The model under review builds one solid part; all positions refer to its coordinate system, in mm. A direction names the side the tool comes from. Coordinates: 2 decimals unless noted, no trailing zeros. Loops run counter-clockwise (first coordinate to the right, second up) from the corner with the lowest first, then second, coordinate; pieces in that order, holes last. Notation, with made-up numbers: (55, -37.75) - (95, -37.75) arc R20 cw to (95, -30.75) - close; hole circle Ø4 at (69, -3.5). An arc over 180 degrees is marked (long way). Use a Markdown table: item, result. Add a question column.
1) Clearance check with flat-ended pins moving along their axes: pin 1 (1.5 mm diameter, centred on x = -10, y = 22, fed in from +Z); pin 2 (2 mm diameter, centred on y = 10, z = 2, fed in from -X); pin 3 (3 mm diameter, centred on x = -2, z = 0.5, fed in from -Y). State where each tip first meets the part, or that it passes through.
2) The part is to be moulded in two halves that separate along X. For faces 4 (the cylindrical face through (-3, 0, 4)), 5 (the cylindrical face through (1.27, -0.97, 0.99)), 6 (the flat face through (2, 16, 4)), 7 (the cylindrical face through (-12, 24, 1)), say which applies: pulls with the +X half, pulls with the -X half, needs draft (parallel to the pull), parting line crosses it, or undercut.
3) Add section A-A, the plane y = 21. Give the boundary of the cut face in (x, z), and give its area (3 significant figures).
4) Add section B-B, the plane x = 0. Give the boundary of the cut face in (y, z), and give its area (3 significant figures).
5) Add section C-C, the plane z = 1.6. Give the boundary of the cut face in (x, y).
6) Add section D-D, the plane y = 0. Give the boundary of the cut face in (x, z), and give its area (3 significant figures).
7) To check wall thickness, follow L1, parallel to Z at x = -4, y = 14.5; L2, parallel to Y at x = -4, z = 2.55; L3, parallel to Y at x = -4.25, z = 0.9. State the ranges of each line that lie inside material, in increasing order. Write a range as [from, to].
8) For faces 1 (the flat face through (-1.3, -1.3, 2)), 2 (the cylindrical face through (6.89, 22.01, 1.48)), 3 (the flat face through (-2, 16, 4)), list the 3-axis set-ups (+Z, -Z, +X, -X, +Y, -Y) from which the entire face can be reached by the end or side of a thin tool; tool diameter is ignored.
```python
from build123d import *
from build123d.topology import SkipClean

# Parameters (mm, degrees)
SZKIC1_R                    = 2.75
SZKIC1_R_2                  = 1.5
DODANIE_WYCI_GNI_CIE1_DEPTH = 3
SZKIC2_R                    = 6.131623165
SZKIC2_R_2                  = 2.75
DODANIE_WYCI_GNI_CIE2_DEPTH = 3
SZKIC3_R                    = 3
SZKIC3_R_2                  = 1.6
DODANIE_WYCI_GNI_CIE3_DEPTH = 2
SZKIC4_W                    = 4
SZKIC4_H                    = 20.653159846
DODANIE_WYCI_GNI_CIE4_DEPTH = 2
SZKIC6_R                    = 3
WYTNIJ_WYCI_GNI_CIE1_DEPTH  = 4


with BuildPart() as part:
    # Szkic1 → Dodanie-wyciągnięcie1 (new body)
    with BuildSketch(Plane.XY):
        with BuildLine():
            Line((-8, 26), (8, 26))
            ThreePointArc((8, 26), (12.044264582, 23.940055101), (12.756144284, 19.457569598))
            Line((12.756144284, 19.457569598), (5.832576894, -1.891520397))
            ThreePointArc((5.832576894, -1.891520397), (0, -6.131623165), (-5.832576894, -1.891520397))
            Line((-5.832576894, -1.891520397), (-12.756144284, 19.457569598))
            ThreePointArc((-12.756144284, 19.457569598), (-12.044264582, 23.940055101), (-8, 26))
        make_face()
        Circle(SZKIC1_R, mode=Mode.SUBTRACT)
        with Locations((8, 21)):
            Circle(SZKIC1_R_2, mode=Mode.SUBTRACT)
        with Locations((-8, 21)):
            Circle(SZKIC1_R_2, mode=Mode.SUBTRACT)
    extrude(amount=DODANIE_WYCI_GNI_CIE1_DEPTH)

    # Szkic2 → Dodanie-wyciągnięcie2 (add)
    with BuildSketch(Plane.XY.offset(3)):
        with Locations(Location((0, 0, 0), (0, 0, 197.968018337))):
            Circle(SZKIC2_R)
        Circle(SZKIC2_R_2, mode=Mode.SUBTRACT)
    extrude(amount=DODANIE_WYCI_GNI_CIE2_DEPTH)

    # Szkic3 → Dodanie-wyciągnięcie3 (add)
    with BuildSketch(Plane(origin=(0, 0, 0), x_dir=(-1, 0, 0), z_dir=(0, 0, -1))):
        Circle(SZKIC3_R)
        Circle(SZKIC3_R_2, mode=Mode.SUBTRACT)
    extrude(amount=-DODANIE_WYCI_GNI_CIE3_DEPTH)

    # Szkic4 → Dodanie-wyciągnięcie4 (add)
    with BuildSketch(Plane.XY.offset(3)):
        with Locations((0, 15.673420077)):
            Rectangle(SZKIC4_W, SZKIC4_H)
    extrude(amount=DODANIE_WYCI_GNI_CIE4_DEPTH)

    # Szkic6 → Wytnij-wyciągnięcie1 (cut)
    with SkipClean():  # the faces are left unmerged after this step: merging them gives an invalid solid
        with BuildSketch(Plane.XY.offset(6)):
            Circle(SZKIC6_R)
        extrude(amount=-WYTNIJ_WYCI_GNI_CIE1_DEPTH, mode=Mode.SUBTRACT)


solid = part.part
```
From the geometry:
| question | item | result |
|---|---|---|
| 1 | pin 1 | stops at z = 3 |
| 1 | pin 2 | stops at x = -10.01 |
| 1 | pin 3 | stops at y = -6.11 |
| 2 | face 4 | undercut |
| 2 | face 5 | undercut |
| 2 | face 6 | pulls with the +X half |
| 2 | face 7 | pulls with the -X half |
| 3 | outline | (-13, 0) - (-9.5, 0) - (-9.5, 3) - (-13, 3) - close; (-6.5, 0) - (6.5, 0) - (6.5, 3) - (2, 3) - (2, 5) - (-2, 5) - (-2, 3) - (-6.5, 3) - close; (9.5, 0) - (13, 0) - (13, 3) - (9.5, 3) - close |
| 3 | area | 68.0 mm^2 |
| 4 | outline | (-6.13, 0) - (-1.6, 0) - (-1.6, 2) - (-3, 2) - (-3, 6) - (-6.13, 6) - close; (1.6, 0) - (26, 0) - (26, 5) - (6.13, 5) - (6.13, 6) - (3, 6) - (3, 2) - (1.6, 2) - close |
| 4 | area | 143 mm^2 |
| 5 | outline | (-12.76, 19.46) - (-5.83, -1.89) arc R6.13 ccw to (5.83, -1.89) - (12.76, 19.46) arc R5 ccw to (8, 26) - (-8, 26) arc R5 ccw to start; hole circle Ø3 at (-8, 21); hole circle Ø3.2 at (0, 0); hole circle Ø3 at (8, 21) |
| 6 | outline | (-6.45, 0) - (-1.6, 0) - (-1.6, 2) - (-3, 2) - (-3, 6) - (-6.13, 6) - (-6.13, 3) - (-6.45, 3) - close; (1.6, 0) - (6.45, 0) - (6.45, 3) - (6.13, 3) - (6.13, 6) - (3, 6) - (3, 2) - (1.6, 2) - close |
| 6 | area | 45.1 mm^2 |
| 7 | L1 | z = [0, 3] |
| 7 | L2 | y = [-4.65, 26] |
| 7 | L3 | y = [-4.42, 26] |
| 8 | face 1 | +Z |
| 8 | face 2 | +Z, -Z |
| 8 | face 3 | +Z, -X, +Y |
